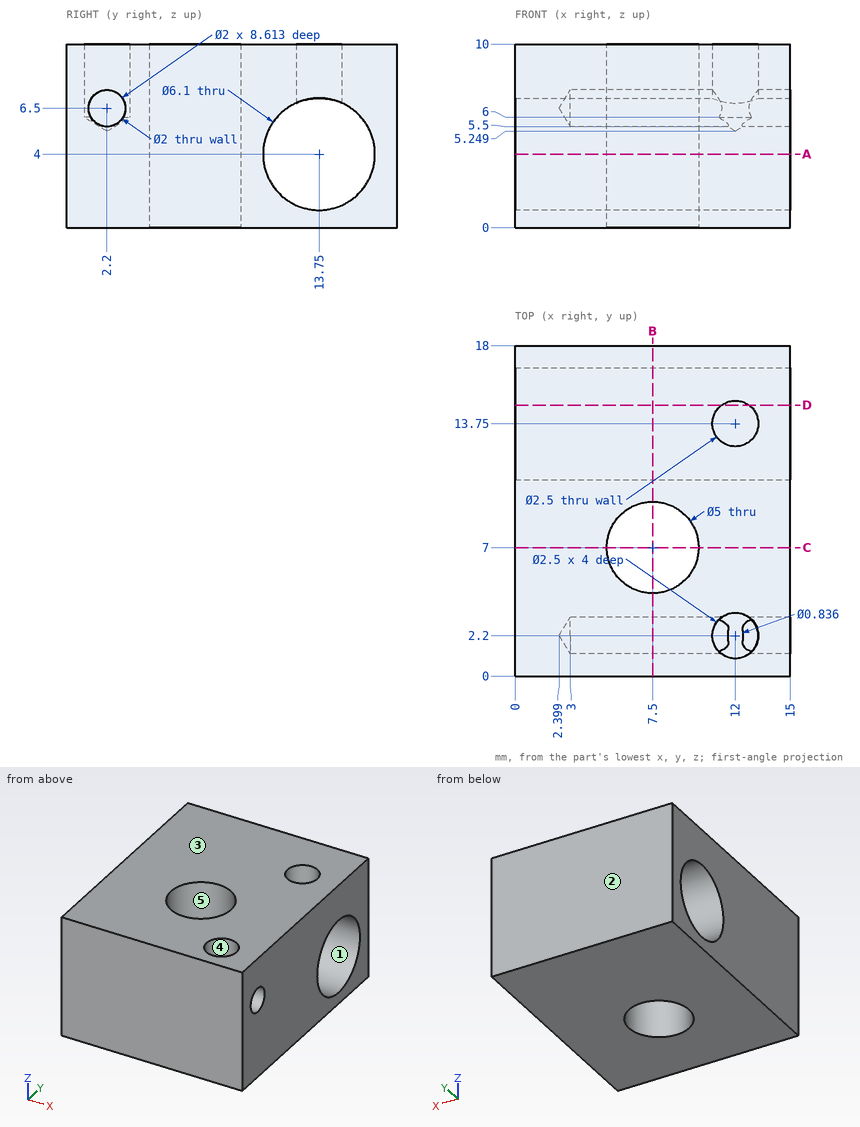
Source: three-view drawing plus pictorial views. Frame: mm from the lowest corner of the part. A direction names the side the tool comes from. Give positions to 0.01 mm unless a question says otherwise; leave off trailing zeros. Order: outer loops, then holes, each group sorted by start corner. A loop starts at its lowest first (then second) coordinate and runs counter-clockwise, first axis right, second up.
1. Section B-B on x = 7.5. Return the cut outline in (y, z).
Derived:
outline: (0, 0) - (4.5, 0) - (4.5, 10) - (0, 10) - close; (9.5, 0) - (18, 0) - (18, 10) - (9.5, 10) - close; hole circle Ø2 at (2.2, 6.5); hole circle Ø6.1 at (13.75, 4)
2. Section A-A on z = 4. Return the cut outline in (x, y).
Derived:
outline: (0, 0) - (15, 0) - (15, 10.7) - (0, 10.7) - close; (0, 16.8) - (15, 16.8) - (15, 18) - (0, 18) - close; hole circle Ø5 at (7.5, 7)
3. Mould query, pull axis Z, two halves, no side actions, for the marked faces 1, 2 and 3. Classes: released by +Z, released by -Z, zero draft, split by the parting line, or undercut.
Derived:
face 1: undercut
face 2: zero draft
face 3: released by +Z
4. Reachability of the marked faces 4 and 5 from +Z, -Z, +X, -X, +Y, -Y: full face, straight path, thin tool, end or side. Return the list, or none.
Derived:
face 4: +Z
face 5: +Z, -Z
5. Pin query (flat end, axial travel): pin 1 (1.2 mm diameter, centred on y = 2.2, z = 6.5, fed in from +X). Return the tip coordinate at first contact, or that it passes through.
Derived:
pin 1: stops at x = 2.76
6. Section C-C on y = 7. Return the cut outline in (x, z), and give its area (3 significant figures).
Derived:
outline: (0, 0) - (5, 0) - (5, 10) - (0, 10) - close; (10, 0) - (15, 0) - (15, 10) - (10, 10) - close
area: 100 mm2
7. Material intervals for L1, parallel to Y at x = 12, z = 8.5; L2, parallel to X at y = 13.75, z = 8.6; L3, parallel to Z at x = 10, y = 2.2, sorted ascending.
Derived:
L1: y = 0 to 0.95, 3.45 to 12.5, 15 to 18
L2: x = 0 to 10.75, 13.25 to 15
L3: z = 0 to 5.5, 7.5 to 10
8. Section D-D on y = 14.75. Return the cut outline in (x, z).
Derived:
outline: (0, 0) - (15, 0) - (15, 1.12) - (0, 1.12) - close; (0, 6.88) - (11.25, 6.88) - (11.25, 10) - (0, 10) - close; (12.75, 6.88) - (15, 6.88) - (15, 10) - (12.75, 10) - close
